Check sheet for the modelled part. Datum: model origin and axes. Units: mm. A direction names the side the tool comes from. Round coordinates to 2 decimals unless told otherwise and drop trailing zeros. Write each loop counter-clockwise with the first axis right and the second up, starting at its lowest first coordinate (ties: lowest second). Pieces come first, ordered by that corner, then holes.
Item 1: Release check for a two-part mould opening along Z. For faces 6 (the flat face through (88, -15.3, 22.5)), 7 (the cylindrical face through (103.7, -14.807, -25.035)), 8 (the flat face through (114.78, -40.05, -32.59)) record: pulls with the +Z half, pulls with the -Z half, needs draft (parallel to the pull), parting line crosses it, or undercut.
Item 2: Set-up check for faces 1 (the flat face through (74, -10, 27.5)), 2 (the flat face through (108.5, -36, 25.4)), 3 (the cylindrical face through (-39.965, -5.369, 17.497)), 4 (the flat face through (-14, -20, 0)), 5 (the cylindrical face through (115.035, -134.511, -39.954)): record each of +Z, -Z, +X, -X, +Y, -Y from which the full face is reachable in a straight line by a thin tool's end or side.
Item 3: Material ranges on line 1 along X through (y, z) = (3.75, -15); line 2 along Z through (x, y) = (70.5, -10.5); line 3 along X through (y, z) = (-12, -24), recorded low to high.
Item 4: Depth check by flat-ended pin: pin 1 (7 mm diameter, centred on x = 102.5, y = -12.5, fed in from -Z); pin 2 (8 mm diameter, centred on y = -76.5, z = -22.5, fed in from -X); pin 3 (12 mm diameter, centred on x = 23.5, z = 20.5, fed in from -Y); pin 4 (3.5 mm diameter, centred on x = -12.5, z = -15, fed in from +Y). Enter the tip coordinate at first touch or a pass-through.
Item 5: Section check B-B, the plane y = -123.5. Record the cut outline in (x, z), plus the area to 3 significant figures.
Item 6: Section check D-D, the plane y = -6. Record the cut outline in (x, z), plus the area to 3 significant figures.
Item 7: Section check C-C, the plane x = 5. Record the cut outline in (y, z).
Item 8: Section check A-A, the plane x = 87.5. Record the cut outline in (y, z).
from build123d import *

# Parameters (mm, degrees)
SKETCH_1_W          = 85
SKETCH_1_H          = 55
EXTRUDE_1_DEPTH     = 5
SKETCH_2_W          = 5
SKETCH_2_H          = 55
EXTRUDE_2_DEPTH     = 20
SKETCH_3_W          = 55
SKETCH_3_H          = 5
EXTRUDE_3_DEPTH     = 75
SKETCH_7_R          = 2.1
CUT_EXTRUDE_1_DEPTH = 5
EXTRUDE_4_DEPTH     = 5
FILLET_1_R          = 4.5
RIB_START           = -5
RIB_1_DEPTH         = 10
EXTRUDE_5_DEPTH     = 5
SKETCH_12_R         = 2.6
CUT_EXTRUDE_2_DEPTH = 5
CHAMFER_1_SIZE      = 10
CHAMFER_2_SIZE      = 10
SKETCH_13_R         = 2.1
CUT_EXTRUDE_3_DEPTH = 5
CHAMFER_3_SIZE      = 10
FILLET_2_R          = 10
FILLET_3_R          = 10
CHAMFER_4_SIZE      = 2


# Read off the part's stored shape, not the designer's step: 筋1
with BuildPart() as part:
    # 草图1 → 凸台-拉伸1 (new body)
    with BuildSketch(Plane(origin=(0, 0, 0), x_dir=(1, 0, 0), z_dir=(0, 1, 0))):
        Rectangle(SKETCH_1_W, SKETCH_1_H)
    extrude(amount=EXTRUDE_1_DEPTH)

    # 草图2 → 凸台-拉伸2 (add)
    with BuildSketch(Plane.XZ):
        with Locations((-40, 0)):
            Rectangle(SKETCH_2_W, SKETCH_2_H)
    extrude(amount=EXTRUDE_2_DEPTH)

    # 草图3 → 凸台-拉伸3 (add)
    with BuildSketch(Plane(origin=(42.5, 0, 0), x_dir=(0, 0, -1), z_dir=(1, 0, 0))):
        with Locations((0, 2.5)):
            Rectangle(SKETCH_3_W, SKETCH_3_H)
    extrude(amount=EXTRUDE_3_DEPTH)

    # 草图7 → 切除-拉伸1 (cut)
    with BuildSketch(Plane(origin=(0, 5, 0), x_dir=(1, 0, 0), z_dir=(0, 1, 0))):
        with Locations(Location((-12.5, 15, 0), (0, 0, 270))):
            Circle(SKETCH_7_R)
        with Locations(Location((12.5, 15, 0), (0, 0, 270))):
            Circle(SKETCH_7_R)
        with Locations(Location((67.5, 15, 0), (0, 0, 270))):
            Circle(SKETCH_7_R)
        with Locations(Location((92.5, 15, 0), (0, 0, 270))):
            Circle(SKETCH_7_R)
        with Locations(Location((92.5, -15, 0), (0, 0, 90))):
            Circle(SKETCH_7_R)
        with Locations(Location((67.5, -15, 0), (0, 0, 90))):
            Circle(SKETCH_7_R)
        with Locations(Location((12.5, -15, 0), (0, 0, 90))):
            Circle(SKETCH_7_R)
        with Locations(Location((-12.5, -15, 0), (0, 0, 90))):
            Circle(SKETCH_7_R)
    extrude(amount=-CUT_EXTRUDE_1_DEPTH, mode=Mode.SUBTRACT)

    # 草图8 → 凸台-拉伸4 (add)
    with BuildSketch(Plane(origin=(117.5, 0, 0), x_dir=(0, 0, -1), z_dir=(1, 0, 0))):
        Polygon((-33.188754566, -145), (-27.5, -145), (27.5, -145), (60.188754566, -145), (57.031110104, -105), (37.540925534, -45), (27.5, -34.959074466), (27.5, -20), (27.5, 0), (-27.5, 0), (-27.5, -20), (-27.5, -34.959074466), (-37.540925534, -45), (-57.031110104, -105), (-60.188754566, -145), (-42.188754566, -145), align=None)
        Polygon((-32.478284562, -136), (-41.478284562, -136), (-39.031110104, -105), (-19.540925534, -45), (-10.540925534, -45), (-30.031110104, -105), align=None, mode=Mode.SUBTRACT)
        Polygon((41.478284562, -136), (32.478284562, -136), (30.031110104, -105), (10.540925534, -45), (19.540925534, -45), (39.031110104, -105), align=None, mode=Mode.SUBTRACT)
    extrude(amount=-EXTRUDE_4_DEPTH)

    # 圆角1
    # the kernel refuses this fillet: 4.5 mm, written as the material it adds along each edge
    with BuildSketch(Plane(origin=(117.5, -45, -19.540925534), x_dir=(0, -0.9510797935163557, -0.30894534527143475), z_dir=(-1, 0, 0)), Plane(origin=(117.5, -45, 19.540925534), x_dir=(0, 0, -1), z_dir=(-1, 0, 0))) as fillet_1_piece_1:
        with BuildLine():
            CenterArc((FILLET_1_R * 0.726600080708, FILLET_1_R), FILLET_1_R, 197.995683599, 72.004316401)
            Line((-FILLET_1_R * 0.224479712809, FILLET_1_R * 0.691054654729), (0, 0))
            Line((0, 0), (FILLET_1_R * 0.726600080708, 0))
        make_face()
    extrude(amount=5)
    with BuildSketch(Plane(origin=(117.5, -45, -10.540925534), x_dir=(0, 0, -1), z_dir=(-1, 0, 0)), Plane(origin=(117.5, -45, 10.540925534), x_dir=(0, -0.9510797935163557, 0.30894534527143513), z_dir=(-1, 0, 0))) as fillet_1_piece_2:
        with BuildLine():
            CenterArc((FILLET_1_R * 1.3762728997, FILLET_1_R), FILLET_1_R, 162.004316401, 107.995683599)
            Line((FILLET_1_R * 0.425193106186, FILLET_1_R * 1.30894534527), (0, 0))
            Line((0, 0), (FILLET_1_R * 1.3762728997, 0))
        make_face()
    extrude(amount=5)
    with BuildSketch(Plane(origin=(117.5, -136, -32.478284562), x_dir=(0, 0.9968986380141637, 0.07869628660556646), z_dir=(-1, 0, 0))) as fillet_1_piece_3:
        with BuildLine():
            CenterArc((FILLET_1_R * 0.924169898787, FILLET_1_R), FILLET_1_R, 184.513632187, 85.486367813)
            Line((-FILLET_1_R * 0.0727287392272, FILLET_1_R * 0.921303713394), (0, 0))
            Line((0, 0), (FILLET_1_R * 0.924169898787, 0))
        make_face()
    extrude(amount=5)
    with BuildSketch(Plane(origin=(117.5, -136, -41.478284562), x_dir=(0, 0.9968986380141637, 0.07869628660556578), z_dir=(-1, 0, 0))) as fillet_1_piece_4:
        with BuildLine():
            CenterArc((FILLET_1_R * 1.08205212192, -FILLET_1_R), FILLET_1_R, 90, 94.513632187)
            Line((FILLET_1_R * 0.085153483909, -FILLET_1_R * 1.07869628661), (0, 0))
            Line((0, 0), (FILLET_1_R * 1.08205212192, 0))
        make_face()
    extrude(amount=5)
    with BuildSketch(Plane(origin=(117.5, -136, 32.478284562), x_dir=(0, 0.9968986380141636, -0.078696286605567), z_dir=(-1, 0, 0))) as fillet_1_piece_5:
        with BuildLine():
            CenterArc((FILLET_1_R * 0.924169898787, -FILLET_1_R), FILLET_1_R, 90, 85.486367813)
            Line((-FILLET_1_R * 0.0727287392272, -FILLET_1_R * 0.921303713394), (0, 0))
            Line((0, 0), (FILLET_1_R * 0.924169898787, 0))
        make_face()
    extrude(amount=5)
    with BuildSketch(Plane(origin=(117.5, -136, 41.478284562), x_dir=(0, 0.9968986380141637, -0.07869628660556578), z_dir=(-1, 0, 0))) as fillet_1_piece_6:
        with BuildLine():
            CenterArc((FILLET_1_R * 1.08205212192, FILLET_1_R), FILLET_1_R, 175.486367813, 94.513632187)
            Line((FILLET_1_R * 0.085153483909, FILLET_1_R * 1.07869628661), (0, 0))
            Line((0, 0), (FILLET_1_R * 1.08205212192, 0))
        make_face()
    extrude(amount=5)

    # 筋1 outline → 筋1 (add)
    with BuildSketch(Plane.XY.offset(RIB_START)):
        Polygon((-37.5, 0), (-37.5, -20), (37.5, -20), (112.5, -95), (112.5, 0), align=None)
    extrude(amount=RIB_1_DEPTH)

    # 草图10 → 凸台-拉伸5 (add)
    with BuildSketch(Plane.XY.offset(27.5)):
        Polygon((112.5, 0), (112.5, -30), (82.5, -30), (52.5, 0), align=None)
    extrude_5 = extrude(amount=-EXTRUDE_5_DEPTH)

    # 草图12 → 切除-拉伸2 (cut)
    with BuildSketch(Plane.XY.offset(27.5)):
        with Locations((87.5, -12.5)):
            Circle(SKETCH_12_R)
        with Locations((102.5, -12.5)):
            Circle(SKETCH_12_R)
    cut_extrude_2 = extrude(amount=-CUT_EXTRUDE_2_DEPTH, mode=Mode.SUBTRACT)

    # 镜向2: 凸台-拉伸5, 切除-拉伸2 across plane
    add(extrude_5.mirror(Plane.XY))
    add(cut_extrude_2.mirror(Plane.XY), mode=Mode.SUBTRACT)

    # 倒角1
    chamfer_1_edges = [part.edges().sort_by_distance(p)[0] for p in [
        (112.5, -30, -25),
        (112.5, -30, 25),
    ]]
    chamfer(chamfer_1_edges, length=CHAMFER_1_SIZE)

    # 倒角2
    chamfer_2_edges = [part.edges().sort_by_distance(p)[0] for p in [
        (112.5, 0, -13.75),
        (112.5, 0, 13.75),
    ]]
    chamfer(chamfer_2_edges, length=CHAMFER_2_SIZE)

    # 草图13 → 切除-拉伸3 (cut)
    with BuildSketch(Plane(origin=(-37.5, 0, 0), x_dir=(0, 0, -1), z_dir=(1, 0, 0))):
        with Locations((-19.5, -6)):
            Circle(SKETCH_13_R)
        with Locations((-13, -14)):
            Circle(SKETCH_13_R)
    cut_extrude_3 = extrude(amount=-CUT_EXTRUDE_3_DEPTH, mode=Mode.SUBTRACT)

    # 镜向3: 切除-拉伸3 across plane
    add(cut_extrude_3.mirror(Plane.XY), mode=Mode.SUBTRACT)

    # 倒角3
    chamfer_3_edges = [part.edges().sort_by_distance(p)[0] for p in [
        (-40, -20, 27.5),
        (-40, -20, -27.5),
    ]]
    chamfer(chamfer_3_edges, length=CHAMFER_3_SIZE)

    # 圆角2
    fillet_2_edges = [part.edges().sort_by_distance(p)[0] for p in [
        (112.5, -95, 0),
        (37.5, -20, 0),
    ]]
    fillet(fillet_2_edges, radius=FILLET_2_R)

    # 圆角3
    fillet_3_edges = [part.edges().sort_by_distance(p)[0] for p in [
        (52.5, 0, 25),
        (52.5, 0, -25),
    ]]
    fillet(fillet_3_edges, radius=FILLET_3_R)

    # 倒角4
    chamfer_4_edges = [part.edges().sort_by_distance(p)[0] for p in [
        (-37.5, 0, -16.25),
        (-37.5, 0, 16.25),
    ]]
    chamfer(chamfer_4_edges, length=CHAMFER_4_SIZE)


solid = part.part
Values found:
1. face 6: undercut
1. face 7: needs draft
1. face 8: pulls with the -Z half
2. face 1: +Z, +X, -X, +Y
2. face 2: +Z, -X, -Y
2. face 3: -X
2. face 4: +Z, -Z, -X, -Y
2. face 5: +X, -X
3. line 1: x = -42.5 to -14.6, -10.4 to 10.4, 14.6 to 65.4, 69.6 to 90.4, 94.6 to 117.5
3. line 2: z = -27.5 to -22.5, -5 to 5, 22.5 to 27.5
3. line 3: x = -42.5 to -37.5, 64.5 to 84.95, 90.05 to 99.95, 105.05 to 117.5
4. pin 1: stops at z = -27.5
4. pin 2: stops at x = 112.5
4. pin 3: stops at y = 0
4. pin 4: passes through
5. outline: (112.5, -58.49) - (117.5, -58.49) - (117.5, -40.49) - (112.5, -40.49) - close; (112.5, -31.49) - (117.5, -31.49) - (117.5, 31.49) - (112.5, 31.49) - close; (112.5, 40.49) - (117.5, 40.49) - (117.5, 58.49) - (112.5, 58.49) - close
5. area: 495 mm2
6. outline: (-42.5, -27.5) - (-37.5, -27.5) - (-37.5, -21.6) - (-42.5, -21.6) - close; (-42.5, -17.4) - (-37.5, -17.4) - (-37.5, -5) - (108.5, -5) - (108.5, -22.5) - (58.5, -22.5) - (58.5, -27.5) - (117.5, -27.5) - (117.5, 27.5) - (58.5, 27.5) - (58.5, 22.5) - (108.5, 22.5) - (108.5, 5) - (-37.5, 5) - (-37.5, 17.4) - (-42.5, 17.4) - close; (-42.5, 21.6) - (-37.5, 21.6) - (-37.5, 27.5) - (-42.5, 27.5) - close
6. area: 2,690 mm2
7. outline: (-20, -5) - (0, -5) - (0, -27.5) - (5, -27.5) - (5, 27.5) - (0, 27.5) - (0, 5) - (-20, 5) - close
8. outline: (-70, -5) - (0, -5) - (0, -22.5) - (-9.9, -22.5) - (-9.9, -27.5) - (5, -27.5) - (5, 27.5) - (-9.9, 27.5) - (-9.9, 22.5) - (0, 22.5) - (0, 5) - (-70, 5) - close; (-30, -27.5) - (-15.1, -27.5) - (-15.1, -22.5) - (-30, -22.5) - close; (-30, 22.5) - (-15.1, 22.5) - (-15.1, 27.5) - (-30, 27.5) - close
